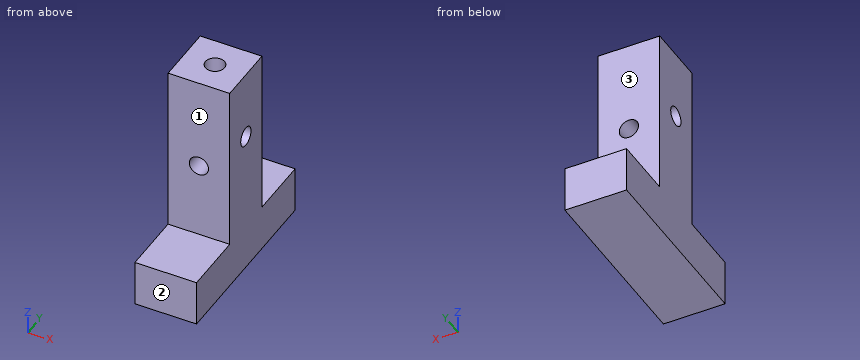
Autodesk Inventor part; units mm, degrees
ref_plane "YZ Plane" through (0, 0, 0) normal (1, 0, 0) x (0, 1, 0)
ref_plane "XZ Plane" through (0, 0, 0) normal (0, 1, 0) x (-1, 0, 0)
ref_plane "XY Plane" through (0, 0, 0) normal (0, 0, 1) x (1, 0, 0)
sketch "Sketch1" plane through (0, 0, 0) normal (0, 0, 1) x (1, 0, 0)
  line L0 (-6.35, -19.05) -> (6.35, -19.05)
  line L1 (6.35, -19.05) -> (6.35, 19.05)
  line L2 (6.35, 19.05) -> (-6.35, 19.05)
  line L3 (-6.35, 19.05) -> (-6.35, -19.05)
  line L4 (-6.35, -19.05) -> (6.35, 19.05) construction
  line L5 (6.35, -19.05) -> (-6.35, 19.05) construction
  point P0 (0, 0)
  dimension "height" = 38.1
  dimension "width" = 12.7
extrude "Extrusion9" add sketch "Sketch1" against normal blind 9.525
sketch "Sketch19" plane through (0, 0, 0) normal (0, 0, 1) x (1, 0, 0)
  line L0 (-6.35, -6.223) -> (6.35, -6.223)
  line L1 (6.35, -6.223) -> (6.35, 6.223)
  line L2 (6.35, 6.223) -> (-6.35, 6.223)
  line L3 (-6.35, 6.223) -> (-6.35, -6.223)
  line L4 (-6.35, -6.223) -> (6.35, 6.223) construction
  line L5 (6.35, -6.223) -> (-6.35, 6.223) construction
  line L6 (-6.35, 19.05) -> (-6.35, -19.05)
  point P0 (0, 0)
  dimension "d126" = 12.446
extrude "Extrusion10" add sketch "Sketch19" along normal blind 34.798
sketch "Sketch20" plane through (6.35, -19.05, -9.525) normal (1, 0, 0) x (0, 0, -1)
  line L0 (-9.525, 25.273) -> (-9.525, 38.1)
  line L1 (-9.525, 19.05) -> (-44.323, 19.05) construction
  line L2 (-44.323, 25.273) -> (-44.323, 12.827) construction
  point P0 (-30.099, 19.05)
  dimension "d129" = 20.574
  dimension "d137" = 0
hole "Hole13" at (6.35, 0, 20.574) direction (-1, 0, 0) diameter 3.9624 end through all
sketch "Sketch21" plane through (0, 0, 34.798) normal (0, 0, 1) x (1, 0, 0)
  point P0 (0, 0)
  point P1 (0, 0)
hole "Hole14" at (0, 0, 34.798) direction (0, 0, -1) diameter 3.9624 depth 10.16 tip angle 118
sketch "Sketch22" plane through (-6.35, -6.223, 0) normal (0, -1, 0) x (1, 0, 0)
  point P0 (6.35, 0)
sketch "Sketch23" plane through (-6.35, -6.223, 0) normal (0, -1, 0) x (1, 0, 0)
  line L0 (0, 34.798) -> (12.7, 34.798)
  point P0 (6.35, 0)
  point P1 (6.35, 15.748)
  dimension "d145" = 19.05
hole "Hole15" at (0, -6.223, 15.748) direction (0, 1, 0) diameter 3.9624 end through all
equation "\"height\" = partHeight"
equation "\"width\" = partWidth"
equation "\"d124\" = depthBehindPlate"
equation "\"d126\" = slotWidth"
equation "\"d127\" = 2 * centerLineOfCylinder + plateThickness"
equation "\"partWidth\" = 12.7"
equation "\"centerLineOfCylinder\" = 14.224"
equation "\"partHeight\" = 38.1"
equation "\"depthBehindPlate\" = 9.525"
equation "\"plateThickness\" = 6.35"
equation "\"printerOffset\" = 0.254"
properties part number "vexSupportForArm" material "Aluminum 6061"
Input: part model. Units: mm. Frame: model coordinates. Face numbers are marked on the shaded views. A direction names the side the tool comes from. Coordinates: 2 decimals unless noted, no trailing zeros. Order: outer loops, then holes, each group sorted by start corner. A loop starts at its lowest first (then second) coordinate and runs counter-clockwise, first axis right, second up. Notation, with made-up numbers: M 75,70.25 L 81,70.25 A23 cw 81,80.25 Z; hole C 81.25,8 d10. An arc over 180 degrees is marked long. Write item = value, one per line. Start each with the question number.
(1) Section C-C on z = 31. Output: boundary loops of the cut face in (x, y), and give its area (3 significant figures).
(2) Line query: line 1 along X through (y, z) = (0, 28); line 2 along Z through (x, y) = (0, 3) (3 decimals); line 3 along Y through (x, z) = (0, 30). Output: solid intervals per line, ascending. Write a range as [from, to].
(3) Section B-B on z = 14.5. Output: boundary loops of the cut face in (x, y), and give its area (3 significant figures).
(4) Reachability of the marked faces 1, 2 and 3 from +Z, -Z, +X, -X, +Y, -Y: full face, straight path, thin tool, end or side. Return the list, or none.
(5) First-contact query: P1, Ø6.5, axis at x = -1.5, z = 24, coming from the +Y side; P2, Ø4, axis at y = -7, z = 25, coming from the -X side; P3, Ø3, axis at x = 0, y = 0, coming from the +Z side; P4, Ø6.5, axis at x = -0.5, y = -15.5, coming from the +Z side. Flat tips, straight axial feed; report the tip coordinate or a pass-through.
(6) Section D-D on x = 1.5. Give the number of separate pieces and of enclosed holes in the cut face, and give its area (3 significant figures).
(7) Section A-A on x = 4. Output: boundary loops of the cut face in (y, z) (3 decimals), and give its area (3 significant figures).
Result set:
q1.outline = M -6.35,-6.22 L 6.35,-6.22 L 6.35,6.22 L -6.35,6.22 Z; hole C 0,0 d3.96
q1.area = 146 mm²
q2.line_1 = [-6.35, -1.98], [1.98, 6.35]
q2.line_2 = [-9.525, 13.767], [17.729, 34.798]
q2.line_3 = [-6.22, -1.98], [1.98, 6.22]
q3.outline = M -6.35,-6.22 L -1.54,-6.22 L -1.54,6.22 L -6.35,6.22 Z; M 1.54,-6.22 L 6.35,-6.22 L 6.35,6.22 L 1.54,6.22 Z
q3.area = 120 mm²
q4.face_1 = +Z, +X, -X, -Y
q4.face_2 = +Z, -Z, +X, -X, -Y
q4.face_3 = +Z, +X, -X, +Y
q5.P1 = 6.22
q5.P2 = -6.35
q5.P3 = 24.35
q5.P4 = 0
q6.separate_pieces = 2
q6.enclosed_holes = 1
q6.area = 725 mm²
q7.outline = M -19.05,-9.525 L 19.05,-9.525 L 19.05,0 L 6.223,0 L 6.223,34.798 L -6.223,34.798 L -6.223,0 L -19.05,0 Z; hole C 0,20.574 d3.962
q7.area = 784 mm²
